Source: CAD feature listing. Evaluate the final solid. Frame: model axes, mm. A direction names the side the tool comes from. Coordinates: 2 decimals unless noted, no trailing zeros. Write each loop counter-clockwise with the first axis right and the second up, starting at its lowest first coordinate (ties: lowest second). Pieces come first, ordered by that corner, then holes. Notation, with made-up numbers: M 31.5,45 L 67.5,45 A16 cw 67.5,75 Z; hole C 48,11.5 d5. An arc over 180 degrees is marked long. Write item = value, one per line. Start each with the question number.
1. Line query: line 1 along X through (y, z) = (26, 0.45). Output: solid intervals per line, ascending.
2. Section query A-A (z = 1.7). Output: boundary loops of the cut face in (x, y), then the cut area to 3 significant figures.
3. Access query for faces 1 (the face through (-2, 25.397, 2)), 2 (the face through (0, 6, 2)), 3 (the face through (111, 33, 2)), 4 (the face through (111, 6, 2)). Directions: +Z, -Z, +X, -X, +Y, -Y. A direction counts if a zero-diameter tool reaches every point of the face in a straight line with its end or side. Return the directions, or none.
4. Pin query (flat end, axial travel): pin 1 Ø2 at (y, z) = (27, 3.5) entering from +X; pin 2 Ø2.5 at (x, z) = (-1.5, 2.5) entering from +Y; pin 3 Ø2 at (x, z) = (82, 1) entering from -Y; pin 4 Ø2.5 at (y, z) = (31.5, 3) entering from -X. Return the tip coordinate at first contact, or that it passes through.
5. Section query B-B (y = 2.5). Output: boundary loops of the cut face in (x, z).
```python
from build123d import *

# Parameters (mm, degrees)
CROQUIS1_W              = 111
CROQUIS1_H              = 40
SALIENTE_EXTRUIR1_DEPTH = 5
CROQUIS2_W              = 5
CROQUIS2_H              = 13.333333333
SALIENTE_EXTRUIR2_DEPTH = 5
CROQUIS3_W              = 5
CROQUIS3_H              = 13.333333333
SALIENTE_EXTRUIR3_DEPTH = 5


with BuildPart() as part:
    # Croquis1 → Saliente-Extruir1 (new body)
    with BuildSketch(Plane.XY):
        with Locations((55.5, 20)):
            Rectangle(CROQUIS1_W, CROQUIS1_H)
    extrude(amount=SALIENTE_EXTRUIR1_DEPTH)

    # Croquis2 → Saliente-Extruir2 (add)
    with BuildSketch(Plane(origin=(111, 0, 0), x_dir=(0, 0, -1), z_dir=(1, 0, 0))):
        with Locations((-2.5, 18.729999967)):
            Rectangle(CROQUIS2_W, CROQUIS2_H)
    extrude(amount=SALIENTE_EXTRUIR2_DEPTH)

    # Croquis3 → Saliente-Extruir3 (add)
    with BuildSketch(Plane.ZY):
        with Locations((2.5, 18.729999967)):
            Rectangle(CROQUIS3_W, CROQUIS3_H)
    extrude(amount=SALIENTE_EXTRUIR3_DEPTH)


solid = part.part
```
Results are:
q1.line_1 = 0 to 111
q2.outline = M -5,12.06 L 0,12.06 L 0,0 L 111,0 L 111,12.06 L 116,12.06 L 116,25.4 L 111,25.4 L 111,40 L 0,40 L 0,25.4 L -5,25.4 Z
q2.area = 4,570 mm^2
q3.face_1 = +Z, -Z, -X, +Y
q3.face_2 = +Z, -Z, -X, -Y
q3.face_3 = +Z, -Z, +X, +Y
q3.face_4 = +Z, -Z, +X, -Y
q4.pin_1 = 111
q4.pin_2 = 25.4
q4.pin_3 = 0
q4.pin_4 = 0
q5.outline = M 0,0 L 111,0 L 111,5 L 0,5 Z
